Part model, mm, in its own coordinate system. A direction names the side the tool comes from. Coordinates: 2 decimals unless noted, no trailing zeros. Loops run counter-clockwise (first coordinate to the right, second up) from the corner with the lowest first, then second, coordinate; pieces in that order, holes last. Notation, with made-up numbers: (21.5, 58) -> (73.5, 58) arc R15 cw to (73.5, 72) -> close; hole circle Ø3 at (57.25, 44). An arc over 180 degrees is marked (long way). Use one line per item in the form item = value. Start each with the question number.
(1) Band-saw the part on B-B on x = 17. Give the cut face in (y, z).
(2) Drill centre lines: L1, parallel to Y at x = 3.55, z = 0; L2, parallel to Y at x = 17.1, z = 0. Where is each one in solid material? Low to high. Write a range as [from, to].
(3) Band-saw the part on A-A on z = 0. Give the cut face in (x, y), then the cut area to 3 significant figures.
(4) Pin check, flat tips, straight feed: P1, Ø3, axis at x = 10, z = 8, coming from the -Y side; P2, Ø12, axis at y = -5, z = -1.5, coming from the -X side; P3, Ø8, axis at x = 7.5, z = 14, coming from the -Y side; P4, Ø1, axis at x = 11, z = -8, coming from the +Y side. Stop position of each tip, or through.
(5) Band-saw the part on D-D on x = 12.5. Give the cut face in (y, z), then the cut area to 3 significant figures.
(6) 3-axis set-ups, long thin cutter, end or side, ignore diameter. For faces 1 (the flat face through (10, 0, 0)), 2 (the flat face through (7, 0, 0)), 3 (the cylindrical face through (2.784, -1.062, -0.44)): which of +Z, -Z, +X, -X, +Y, -Y reach the whole face in a straight line?
(7) Mould opens along Z. For faces 4 (the cylindrical face through (9.888, -4.336, 19.524)), 5 (the conical face through (8.99, 6.55, 2.72)), 6 (the flat face through (0, 0, 4)) say: +Z half, -Z half, draft (parallel to the pull), parting line (faces both ways), or undercut.
```python
from build123d import *

# Parameters (mm, degrees)
F2_R     = 1.15
F3_DEPTH = 25
F4_R     = 2
F7_R     = 6.5
F7_R_2   = 1.15
F8_DEPTH = 3
F9_R     = 1


with BuildPart() as f1:
    # F0 (on Top) → F1 (revolve)
    with BuildSketch(Plane.XY):
        Polygon((0, 20), (0, 0), (5, 0), (14, 16), (20, 16), (20, 20), align=None)
    revolve(axis=Axis((2.5, 0, 0), (-1, 0, 0)))

    # F2 (on face) → F3 (cut)
    with BuildSketch(Plane(origin=(0, 0, 0), x_dir=(0, -1, 0), z_dir=(-1, 0, 0))):
        Circle(F2_R)
    extrude(amount=-F3_DEPTH, mode=Mode.SUBTRACT)

    # F4
    f4_edges = [f1.edges().sort_by_distance(p)[0] for p in [
        (20, -20, 0),
        (0, -20, 0),
    ]]
    fillet(f4_edges, radius=F4_R)

    # F7 (on offset) → F8 (join)
    with BuildSketch(Plane.YZ.offset(7)):
        Circle(F7_R)
        Circle(F7_R_2, mode=Mode.SUBTRACT)
        Circle(F7_R_2)
    extrude(amount=F8_DEPTH)

    # F9
    f9_edges = [f1.edges().sort_by_distance(p)[0] for p in [
        (10, -6.5, 0),
    ]]
    fillet(f9_edges, radius=F9_R)


solid = f1.part
```
A:
q1.outline = circle Ø40 at (0, 0); hole circle Ø32 at (0, 0)
q2.L1 = [-20, -1.15], [1.15, 20]
q2.L2 = [-20, -16], [16, 20]
q3.outline = (0, -18) arc R2 ccw to (2, -20) -> (18, -20) arc R2 ccw to (20, -18) -> (20, -16) -> (14, -16) -> (8.66, -6.5) -> (9, -6.5) arc R1 ccw to (10, -5.5) -> (10, 5.5) arc R1 ccw to (9, 6.5) -> (8.66, 6.5) -> (14, 16) -> (20, 16) -> (20, 18) arc R2 ccw to (18, 20) -> (2, 20) arc R2 ccw to (0, 18) -> (0, 1.15) -> (5.65, 1.15) -> (7, 3.56) -> (7, -3.56) -> (5.65, -1.15) -> (0, -1.15) -> close
q3.area = 482 mm²
q4.P1 = -18.91
q4.P2 = 0
q4.P3 = -17.32
q4.P4 = 18.54
q5.outline = circle Ø40 at (0, 0); hole circle Ø26.67 at (0, 0)
q5.area = 698 mm²
q6.face_1 = +X
q6.face_2 = none
q6.face_3 = -X
q7.face_4 = parting line
q7.face_5 = undercut
q7.face_6 = draft
